Part model, mm, in its own coordinate system. Face numbers are marked on the shaded views. Round coordinates to 2 decimals unless told otherwise and drop trailing zeros. Loops run counter-clockwise (first coordinate to the right, second up) from the corner with the lowest first, then second, coordinate; pieces in that order, holes last.
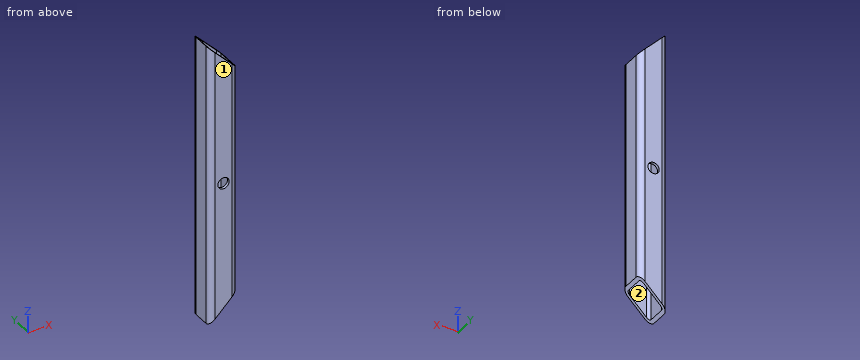
Autodesk Inventor part; units mm, degrees
ref_plane "Piano iniziale" through (0, 0, 0) normal (0, 0, 1) x (1, 0, 0)
ref_plane "Piano finale" through (0, 0, 200) normal (0, 0, 1) x (1, 0, 0)
ref_plane "YZ Plane" through (0, 0, 0) normal (1, 0, 0) x (0, 1, 0)
ref_plane "Piano iniziale" through (0, 0, 0) normal (0, 0, 1) x (1, 0, 0)
ref_plane "Piano finale" through (0, 0, 200) normal (0, 0, 1) x (1, 0, 0)
sketch "Schizzo" plane through (0, 0, 0) normal (0, 0, 1) x (1, 0, 0)
  line L0 (-10, -6) -> (-10, 6)
  line L1 (-6, 10) -> (6, 10)
  line L2 (10, 6) -> (10, -6)
  line L3 (6, -10) -> (-6, -10)
  arc A0 (-10, -6) -> (-6, -10) centre (-6, -6) ccw
  arc A1 (10, 6) -> (6, 10) centre (6, 6) ccw
  arc A2 (-6, 10) -> (-10, 6) centre (-6, 6) ccw
  arc A3 (6, -10) -> (10, -6) centre (6, -6) ccw
  arc A4 (-6, 8) -> (-8, 6) centre (-6, 6) ccw
  line L4 (-6, 8) -> (6, 8)
  arc A5 (8, 6) -> (6, 8) centre (6, 6) ccw
  line L5 (8, 6) -> (8, -6)
  arc A6 (6, -8) -> (8, -6) centre (6, -6) ccw
  line L6 (6, -8) -> (-6, -8)
  arc A7 (-8, -6) -> (-6, -8) centre (-6, -6) ccw
  line L7 (-8, -6) -> (-8, 6)
  line L8 (0, 15.1598) -> (0, -15.1598) construction
  line L9 (-15.1598, 0) -> (15.1598, 0) construction
  dimension "d7" = 4
  dimension "d9" = 20
  dimension "d11" = 20
  dimension "d12" = 2
  dimension "d15" = 10
  dimension "d16" = 10
extrude "Corpo" add sketch "Schizzo" along normal up to surface (200 mm away) from surface at 0
sketch "Sketch3" plane through (0, 0, 0) normal (0, 0, 1) x (1, 0, 0)
  line L0 (0, 0) -> (10, 0)
ref_plane "Work Plane3" through (0, 0, 0) normal (0, -1, 0) x (1, 0, 0)
sketch "Sketch4" plane through (0, 0, 0) normal (0, -1, 0) x (1, 0, 0)
  line L0 (-2, 0) -> (12, 0)
  line L1 (-2, 200) -> (12, 200)
  dimension "d18" = 200
sketch "Schizzo5" plane through (-6, -10, 0) normal (0, -1, 0) x (1, 0, 0)
  line L0 (-4, 0) -> (0, 0)
  line L1 (-4, 0) -> (27.2685, 31.2685)
  line L2 (-4, 0) -> (40.2203, 0) construction
  line L3 (27.2685, 31.2685) -> (27.2685, 0)
  line L4 (27.2685, 0) -> (-4, 0)
  line L5 (-4, 200) -> (31.4981, 164.5019)
  line L6 (-4, 200) -> (46.2019, 200) construction
  line L7 (31.4981, 164.5019) -> (31.4981, 200)
  line L8 (31.4981, 200) -> (-4, 200)
  point P0 (6, 0)
  dimension "d19" = 45
  dimension "d20" = 45
extrude "Estrusione2" cut sketch "Schizzo5" against normal up to next
sketch "Schizzo6" plane through (-6, 10, 196) normal (0, 1, 0) x (1, 0, 0)
  line L0 (12, 180) -> (0, 192)
  line L1 (16, 176) -> (16, 16)
  point P0 (6, 196)
  point P1 (6, 96)
  point P2 (6, 186)
  point P3 (16, 96)
hole "Foro1" at (0, 10, 100) direction (0, -1, 0) diameter 8 end through all
equation "\"d7\" = G_IR"
equation "\"d9\" = G_W"
equation "\"d11\" = G_H"
equation "\"d12\" = G_T"
equation "\"d15\" = 0.5 * d9"
equation "\"d16\" = 0.5 * d11"
equation "\"d3\" = G_L"
equation "\"G_W\" = 20"
equation "\"G_H\" = 20"
equation "\"G_T\" = 2"
equation "\"G_IR\" = 4"
equation "\"G_L\" = d18"
equation "\"G_OFFSET_START\" = 0"
equation "\"G_OFFSET_END\" = 0"
properties part number "ISO 10799-2 - 20x20x2 - 200" material "Acciaio, Dolce"
1) Mould opens along X. For the marked faces 1 and 2 say: released by +X, released by -X, zero draft, split by the parting line, or undercut.
Values:
face 1: zero draft
face 2: undercut
2) Wall check: line 1 along Y through (x, z) = (2, 144); line 2 along X through (y, z) = (-9.45, 100). Give the ranges that are in metal, low to high.
Values:
line 1: y = -10 to -8, 8 to 10
line 2: x = -8.02 to -4, 4 to 8.02
3) Slice it at B-B, the plane z = 100. Give the cut face in (x, y), then the cut area to 3 significant figures.
Values:
outline: (-10, -6) arc R4 ccw to (-6, -10) - (-4, -10) - (-4, -8) - (-6, -8) arc R2 cw to (-8, -6) - (-8, 6) arc R2 cw to (-6, 8) - (-4, 8) - (-4, 10) - (-6, 10) arc R4 ccw to (-10, 6) - close; (4, -10) - (6, -10) arc R4 ccw to (10, -6) - (10, 6) arc R4 ccw to (6, 10) - (4, 10) - (4, 8) - (6, 8) arc R2 cw to (8, 6) - (8, -6) arc R2 cw to (6, -8) - (4, -8) - close
area: 102 mm2
4) Slice it at A-A, the plane y = -0.75. Give the cut face in (x, z).
Values:
outline: (-10, 0) - (-8, 2) - (-8, 198) - (-10, 200) - close; (8, 18) - (10, 20) - (10, 180) - (8, 182) - close
5) Slice it at C-C, the plane x = 0. Give the cut face in (y, z).
Values:
outline: (-10, 10) - (-8, 10) - (-8, 96) - (-10, 96) - close; (-10, 104) - (-8, 104) - (-8, 190) - (-10, 190) - close; (8, 10) - (10, 10) - (10, 96) - (8, 96) - close; (8, 104) - (10, 104) - (10, 190) - (8, 190) - close
6) Slice it at D-D, the plane z = 136. Give the cut face in (x, y).
Values:
outline: (-10, -6) arc R4 ccw to (-6, -10) - (6, -10) arc R4 ccw to (10, -6) - (10, 6) arc R4 ccw to (6, 10) - (-6, 10) arc R4 ccw to (-10, 6) - close; hole (-8, -6) arc R2 ccw to (-6, -8) - (6, -8) arc R2 ccw to (8, -6) - (8, 6) arc R2 ccw to (6, 8) - (-6, 8) arc R2 ccw to (-8, 6) - close
